Check sheet for the modelled part. Datum: model origin and axes. Units: mm. Face numbers are marked on the shaded views. A direction names the side the tool comes from. Coordinates: 2 decimals unless noted, no trailing zeros. Loops run counter-clockwise (first coordinate to the right, second up) from the corner with the lowest first, then second, coordinate; pieces in that order, holes last. Notation, with made-up numbers: (17.25, 0.25) - (50.25, 0.25) arc R27 cw to (50.25, 39.25) - close; hole circle Ø9 at (35, 38). An arc over 180 degrees is marked (long way). Write each question's results on one line, items separated by ' | '. Start each with the question number.
1. Thickness scan on line 1 (X direction, y = 5, z = -26); line 2 (X direction, y = 25, z = -6). Record the ranges inside material, lowest first. Write a range as [from, to].
2. Gauge pin test, flat end, axial feed: P1, Ø10, axis at x = -52, y = -40.5, coming from the +Z side. Record the tip position at first contact, or that the pin passes through.
3. Tool access check on the marked faces 1, 2 and 3. Record the directions out of +Z, -Z, +X, -X, +Y, -Y that give a thin tool (end or side, any length) a straight path to the whole face; none if there is none.
4. Cross-section at C-C (z = -29). Record the cut outline in (x, y), and give its area (3 significant figures).
5. Draft check along Y on the marked faces 4, 5, 6 and 7. Enter one of: released by +Y, released by -Y, zero draft, split by the parting line, or undercut.
6. Cross-section at A-A (y = 23.5). Record the cut outline in (x, z), and give its area (3 significant figures).
7. Cross-section at D-D (z = -8). Record the cut outline in (x, y).
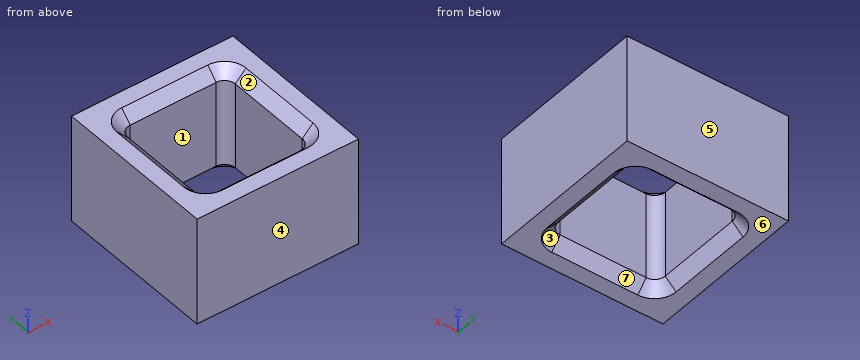
```python
from build123d import *

# Parameters (mm, degrees)
F0_W     = 150
F0_H     = 150
F1_DEPTH = 100
F2_SIZE  = 10
F3_SIZE  = 10


with BuildPart() as f1:
    # F0 (on Top) → F1 (new body)
    with BuildSketch(Plane.XY):
        Rectangle(F0_W, F0_H)
        with BuildLine():
            ThreePointArc((50, -40), (47.071068, -47.071068), (40, -50))
            Line((40, -50), (-40, -50))
            ThreePointArc((-40, -50), (-47.071068, -47.071068), (-50, -40))
            Line((-50, -40), (-50, 40))
            ThreePointArc((-50, 40), (-47.071068, 47.071068), (-40, 50))
            Line((-40, 50), (40, 50))
            ThreePointArc((40, 50), (47.071068, 47.071068), (50, 40))
            Line((50, 40), (50, -40))
        make_face(mode=Mode.SUBTRACT)
    extrude(amount=-F1_DEPTH)

    # F2
    f2_edges = [f1.edges().sort_by_distance(p)[0] for p in [
        (-50, 0, 0),
    ]]
    chamfer(f2_edges, length=F2_SIZE)

    # F3
    f3_edges = [f1.edges().sort_by_distance(p)[0] for p in [
        (50, 0, -100),
    ]]
    chamfer(f3_edges, length=F3_SIZE)


solid = f1.part
```
Established:
1) line 1: [-75, -50], [50, 75] | line 2: [-75, -54], [54, 75]
2) P1: z = -2.99
3) face 1: +Z, -Z | face 2: +Z | face 3: -Z
4) outline: (-75, -75) - (75, -75) - (75, 75) - (-75, 75) - close; hole (-50, -40) arc R10 ccw to (-40, -50) - (40, -50) arc R10 ccw to (50, -40) - (50, 40) arc R10 ccw to (40, 50) - (-40, 50) arc R10 ccw to (-50, 40) - close | area: 12,600 mm^2
5) face 4: released by -Y | face 5: released by +Y | face 6: zero draft | face 7: undercut
6) outline: (-75, -100) - (-60, -100) - (-50, -90) - (-50, -10) - (-60, 0) - (-75, 0) - close; (50, -90) - (60, -100) - (75, -100) - (75, 0) - (60, 0) - (50, -10) - close | area: 4,800 mm^2
7) outline: (-75, -75) - (75, -75) - (75, 75) - (-75, 75) - close; hole (-52, -40) arc R12 ccw to (-40, -52) - (40, -52) arc R12 ccw to (52, -40) - (52, 40) arc R12 ccw to (40, 52) - (-40, 52) arc R12 ccw to (-52, 40) - close
